Can you work these out from the model? Positions are in its coordinate system, mm. Face numbers are marked on the shaded views. A direction names the side the tool comes from. Give positions to 0.01 mm unless a question says otherwise; leave off trailing zeros. Order: outer loops, then holes, each group sorted by start corner. A loop starts at its lowest first (then second) coordinate and runs counter-clockwise, first axis right, second up. Notation, with made-up numbers: (19.5, 57) - (55.5, 57) arc R23 cw to (55.5, 84) - close; hole circle Ø8 at (-39.75, -26). An arc over 180 degrees is marked (long way). Use one line per item in the form item = value. Start each with the question number.
1) Suppose I cut it at D-D, the plane x = 19.75. Write out the boundary of the cut face in (y, z).
2) Please list where these lines run through material, in increasing order: probe 1 along Y at (x, z) = (11.25, 0.9); probe 2 along X at (y, z) = (7.5, 2.75); probe 3 along Y at (x, z) = (16, 11).
3) Suppose I cut it at A-A, the plane z = 1.5. Write out the boundary of the cut face in (x, y), and give its area (3 significant figures).
4) We'd pull the mould along X, two halves only. Please class the marked faces 5, 6 and 7: released by +X, released by -X, zero draft, split by the parting line, or undercut.
5) Suppose I cut it at B-B, the plane y = 5. Write out the boundary of the cut face in (x, z).
6) Suppose I cut it at C-C, the plane x = 11.25. Write out the boundary of the cut face in (y, z).
7) For pin 1 (4.5 mm diameter, centred on y = 4, z = 11, fed in from -X); pin 2 (0.8 mm diameter, centred on y = 5, z = 1.5, fed in from +X); pin 3 (3.5 mm diameter, centred on x = 3, z = 10, fed in from -Y); pin 4 (10 mm diameter, centred on x = 13, z = 13, fed in from +Y), each with a flat end and sliding along its axis, tell me the tip position at first contact or that it passes through.
8) Which directions (+Z, -Z, +X, -X, +Y, -Y) give clear straight access to the entire face, cutting with the end or side of a thin tool? Please do the marked faces 1, 2, 3 and 4.
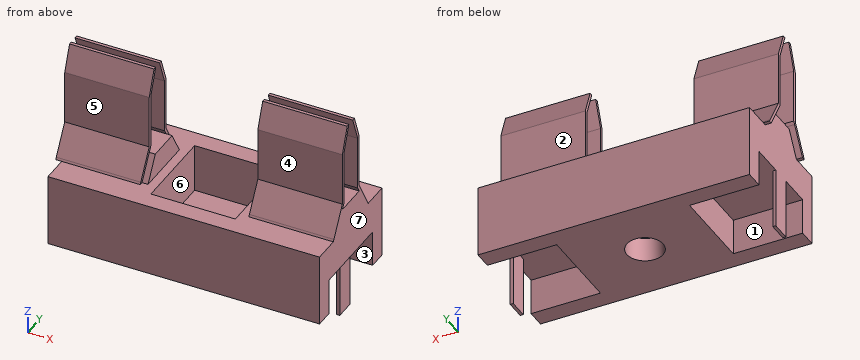
```python
from build123d import *

# Parameters (mm, degrees)
SKETCH_1_W          = 22.5
SKETCH_1_H          = 10
EXTRUDE_1_DEPTH     = 6
SKETCH_2_R          = 1.5
CUT_EXTRUDE_1_DEPTH = 26.342651795
SKETCH_3_W          = 5.75
SKETCH_3_H          = 7
CUT_EXTRUDE_2_DEPTH = 3
CUT_EXTRUDE_3_DEPTH = 4
SKETCH_5_W          = 7
SKETCH_5_H          = 5
EXTRUDE_2_DEPTH     = 2
CUT_EXTRUDE_4_DEPTH = 26.889186932
EXTRUDE_3_DEPTH     = 7
EXTRUDE_4_DEPTH     = 5


with BuildPart() as part:
    # 草图1 → 凸台-拉伸1 (new body)
    with BuildSketch(Plane.XY):
        with Locations((11.25, 5)):
            Rectangle(SKETCH_1_W, SKETCH_1_H)
    extrude(amount=EXTRUDE_1_DEPTH)

    # 草图2 → 切除-拉伸1 (cut, through all)
    with BuildSketch(Plane(origin=(0, 0, 0), x_dir=(-1, 0, 0), z_dir=(0, 0, -1))):
        with Locations((-11.25, 5)):
            Circle(SKETCH_2_R)
    extrude(amount=-CUT_EXTRUDE_1_DEPTH, mode=Mode.SUBTRACT)

    # 草图3 → 切除-拉伸2 (cut)
    with BuildSketch(Plane(origin=(0, 0, 0), x_dir=(-1, 0, 0), z_dir=(0, 0, -1))):
        with Locations((-19.625, 5)):
            Rectangle(SKETCH_3_W, SKETCH_3_H)
        with Locations((-2.875, 5)):
            Rectangle(SKETCH_3_W, SKETCH_3_H)
    extrude(amount=-CUT_EXTRUDE_2_DEPTH, mode=Mode.SUBTRACT)

    # 草图4 → 切除-拉伸3 (cut)
    with BuildSketch(Plane.XY.offset(6)):
        Polygon((14.75, 1.5), (14.75, 8.5), (11.25, 8.5), (7.75, 8.5), (7.75, 1.5), (11.25, 1.5), align=None)
    extrude(amount=-CUT_EXTRUDE_3_DEPTH, mode=Mode.SUBTRACT)

    # 草图5 → 凸台-拉伸2 (add)
    with BuildSketch(Plane.XY.offset(6)):
        with Locations((19, 5)):
            Rectangle(SKETCH_5_W, SKETCH_5_H)
        with Locations((3.5, 5)):
            Rectangle(SKETCH_5_W, SKETCH_5_H)
    extrude(amount=EXTRUDE_2_DEPTH)

    # 草图6 → 切除-拉伸4 (cut, through all)
    with BuildSketch(Plane(origin=(22.5, 0, 0), x_dir=(0, 0, -1), z_dir=(1, 0, 0))):
        Polygon((-6, 7.5), (-8, 6.345299462), (-8, 7.5), align=None)
        Polygon((-8, 3.654700538), (-8, 2.5), (-6, 2.5), align=None)
    extrude(amount=-CUT_EXTRUDE_4_DEPTH, mode=Mode.SUBTRACT)

    # 草图7 → 凸台-拉伸3 (add)
    with BuildSketch(Plane(origin=(22.5, 0, 0), x_dir=(0, 0, -1), z_dir=(1, 0, 0))):
        Polygon((-6, 7.5), (-8.178644615, 6.237293765), (-8.415528154, 6.1), (-12.880891483, 6.1), (-15, 5.308736783), (-15, 5.575596223), (-12.926043311, 6.35), (-8.488722342, 6.35), (-6.157893093, 7.700909921), (-6, 7.792422136), align=None)
        Polygon((-6, 2.5), (-8.178644615, 3.762706235), (-8.415528154, 3.9), (-12.880891483, 3.9), (-15, 4.691263217), (-15, 4.424403777), (-12.926043311, 3.65), (-8.488722342, 3.65), (-6.157893093, 2.299090079), (-6, 2.207577864), align=None)
    extrude_3 = extrude(amount=-EXTRUDE_3_DEPTH)

    # 镜向1: 凸台-拉伸3 across plane
    add(extrude_3.mirror(Plane(origin=(11, 0, 0), x_dir=(0, 0, 1), z_dir=(1, 0, 0))))

    # 草图8 → 凸台-拉伸4 (add)
    with BuildSketch(Plane(origin=(0, 0, 3), x_dir=(-1, 0, 0), z_dir=(0, 0, -1))):
        Polygon((-0.25, 5.8), (-0.25, 5), (0, 5), (0, 5.007441817), (0, 5.8), align=None)
        Polygon((0, 5), (-0.25, 5), (-0.25, 4.2), (0, 4.2), (0, 4.992558183), align=None)
    extrude_4 = extrude(amount=EXTRUDE_4_DEPTH)

    # 镜向2: 凸台-拉伸4 across plane
    add(extrude_4.mirror(Plane(origin=(11, 0, 0), x_dir=(0, 0, 1), z_dir=(1, 0, 0))))


solid = part.part
```
Result sheet:
q1.outline = (0, 0) - (1.5, 0) - (1.5, 3) - (8.5, 3) - (8.5, 0) - (10, 0) - (10, 6) - (7.79, 6) - (6.35, 8.49) - (6.35, 12.93) - (5.58, 15) - (5.31, 15) - (6.1, 12.88) - (6.1, 8.42) - (6.34, 8) - (3.66, 8) - (3.9, 8.42) - (3.9, 12.88) - (4.69, 15) - (4.42, 15) - (3.65, 12.93) - (3.65, 8.49) - (2.21, 6) - (0, 6) - close
q2.probe_1 = 0 to 3.5, 6.5 to 10
q2.probe_2 = 5.75 to 7.75, 14.75 to 16.75
q2.probe_3 = 3.65 to 3.9, 6.1 to 6.35
q3.outline = (0, 0) - (22.5, 0) - (22.5, 1.5) - (16.75, 1.5) - (16.75, 8.5) - (22.5, 8.5) - (22.5, 10) - (0, 10) - (0, 8.5) - (5.75, 8.5) - (5.75, 1.5) - (0, 1.5) - close; (0, 4.2) - (0.25, 4.2) - (0.25, 5.8) - (0, 5.8) - close; (21.75, 4.2) - (22, 4.2) - (22, 5.8) - (21.75, 5.8) - close; hole circle Ø3 at (11.25, 5)
q3.area = 138 mm²
q4.face_5 = zero draft
q4.face_6 = undercut
q4.face_7 = released by +X
q5.outline = (0, -2) - (0.25, -2) - (0.25, 3) - (5.75, 3) - (5.75, 0) - (9.75, 0) - (9.75, 2) - (7.75, 2) - (7.75, 6) - (7, 6) - (7, 8) - (0, 8) - close; (12.75, 0) - (16.75, 0) - (16.75, 3) - (21.75, 3) - (21.75, -2) - (22, -2) - (22, 3) - (22.5, 3) - (22.5, 8) - (15.5, 8) - (15.5, 6) - (14.75, 6) - (14.75, 2) - (12.75, 2) - close
q6.outline = (0, 0) - (3.5, 0) - (3.5, 2) - (1.5, 2) - (1.5, 6) - (0, 6) - close; (6.5, 0) - (10, 0) - (10, 6) - (8.5, 6) - (8.5, 2) - (6.5, 2) - close
q7.pin_1 = -0.5
q7.pin_2 = 22
q7.pin_3 = 3.51
q7.pin_4 = 6.35
q8.face_1 = -Z, -X
q8.face_2 = +Z, +X, -X, +Y
q8.face_3 = -Z, +X
q8.face_4 = +Z, +X, -X, -Y
